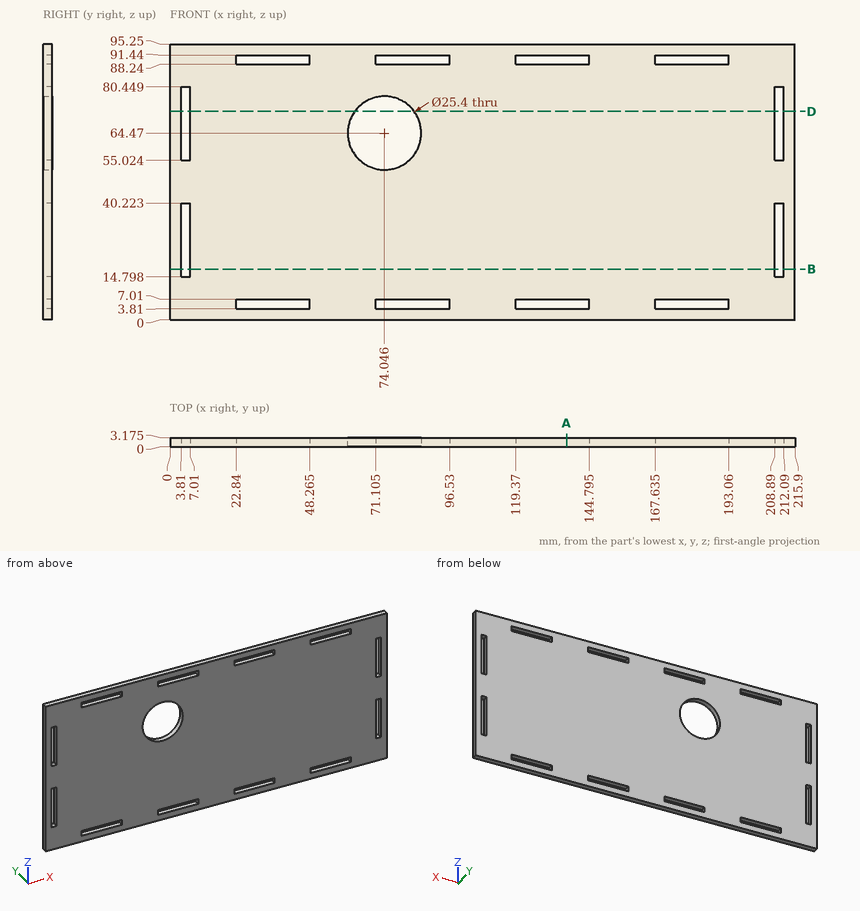
Job drawing, mm, ordinate dimensions from the low corner. One solid piece. Give positions to 0.01 mm unless a question says otherwise; leave off trailing zeros. Loops run counter-clockwise (first coordinate to the right, second up) from the corner with the lowest first, then second, coordinate; pieces in that order, holes last. Notation, with made-up numbers: (71.25, 53.5) - (119.25, 53.5) arc R19 cw to (119.25, 76.5) - close; hole circle Ø3 at (-3.5, -2). An arc over 180 degrees is marked (long way). Use one line per item in the form item = value.
(1) Cut at D-D (z = 72). Give the cut face in (x, y) (1 decimal).
Determined:
outline = (0, 0) - (3.8, 0) - (3.8, 3.2) - (0, 3.2) - close; (7, 0) - (63.8, 0) - (63.8, 3.2) - (7, 3.2) - close; (84.3, 0) - (208.9, 0) - (208.9, 3.2) - (84.3, 3.2) - close; (212.1, 0) - (215.9, 0) - (215.9, 3.2) - (212.1, 3.2) - close
(2) Drop a flat-ended pin along its axis: P1, Ø15, axis at x = 74.05, z = 64.47, coming from the +Y side. Give the stop position or say it passes through.
Determined:
P1 = through
(3) Cut at B-B (z = 17.5). Give the cut face in (x, y) (1 decimal).
Determined:
outline = (0, 0) - (3.8, 0) - (3.8, 3.2) - (0, 3.2) - close; (7, 0) - (208.9, 0) - (208.9, 3.2) - (7, 3.2) - close; (212.1, 0) - (215.9, 0) - (215.9, 3.2) - (212.1, 3.2) - close
(4) Cut at A-A (x = 137). Count the separate pieces of the cut face and the enclosed holes in it, then the cut area to 3 significant figures.
Determined:
separate_pieces = 3
enclosed_holes = 0
area = 282 mm^2
(5) Drill centre lines: L1, parallel to X at y = 1.85, z = 35; L2, parallel to Z at x = 39, y = 1.1; L3, parallel to X at y = 1.3, z = 6.5 (1 decimal). Where is each one in solid material? Low to high.
Determined:
L1 = 0 to 3.81, 7.01 to 208.89, 212.09 to 215.9
L2 = 0 to 3.81, 7.01 to 88.24, 91.44 to 95.25
L3 = 0 to 22.8, 48.3 to 71.1, 96.5 to 119.4, 144.8 to 167.6, 193.1 to 215.9
